```python
from build123d import *

# Parameters (mm, degrees)
SKETCH1_R           = 2.5
BOSS_EXTRUDE1_DEPTH = 8
CHAMFER1_SIZE       = 0.5
SKETCH2_R           = 1.5
CUT_EXTRUDE1_DEPTH  = 5


with BuildPart() as part:
    # Sketch1 → Boss-Extrude1 (new body)
    with BuildSketch(Plane.XY):
        with BuildLine():
            Line((-6, 15), (-6, 0))
            Line((-6, 0), (-25, 0))
            ThreePointArc((-25, 0), (0, -25), (25, 0))
            Line((25, 0), (6, 0))
            Line((6, 0), (6, 15))
            ThreePointArc((6, 15), (0, 21), (-6, 15))
        make_face()
        with Locations((0, 15)):
            Circle(SKETCH1_R, mode=Mode.SUBTRACT)
    extrude(amount=BOSS_EXTRUDE1_DEPTH)

    # Chamfer1
    chamfer1_edges = [part.edges().sort_by_distance(p)[0] for p in [
        (-2.5, 15, 8),
    ]]
    chamfer(chamfer1_edges, length=CHAMFER1_SIZE)

    # Sketch2 → Cut-Extrude1 (cut)
    with BuildSketch(Plane(origin=(0, 21, 0), x_dir=(1, 0, 0), z_dir=(0, 1, 0))):
        with Locations(Location((0, -4, 0), (0, 0, 270))):
            Circle(SKETCH2_R)
    extrude(amount=-CUT_EXTRUDE1_DEPTH, mode=Mode.SUBTRACT)


solid = part.part
```
For this review, take the finished solid that the model builds, in its own axes (mm). A direction names the side the tool comes from. Round coordinates to 2 decimals unless told otherwise and drop trailing zeros. Write each loop counter-clockwise with the first axis right and the second up, starting at its lowest first coordinate (ties: lowest second). Pieces come first, ordered by that corner, then holes. Notation, with made-up numbers: M 22.25,-14 L 60.25,-14 A21 cw 60.25,2 Z; hole C 4.5,-7 d10. An arc over 180 degrees is marked long. One line per item, written item: value. Start each with the question number.
(1) Insertion check: pin 1 (2 mm diameter, centred on x = 12.5, z = 5, fed in from +Y); pin 2 (4 mm diameter, centred on x = 0, z = 4, fed in from +Y); pin 3 (1.5 mm diameter, centred on y = 5.5, z = 5, fed in from +X); pin 4 (3 mm diameter, centred on y = -18.5, z = 1.5, fed in from -X). Each pin has a flat end and moves straight along its axis. Give the tip position at first contact, or say it passes through.
(2) The part is to be moulded in two halves that separate along Z. For faces 4 (the cylindrical face through (-0.575, 19.028, 5.386)), 5 (the flat face through (0, -7, 8)), 6 (the flat face through (-6, 8, 4)), 7 (the flat face through (0, -7, 0)), say which applies: released by +Z, released by -Z, zero draft, split by the parting line, or undercut.
(3) Machinability: for faces 1 (the flat face through (-15, 0, 4)), 2 (the cylindrical face through (-0.54, 12.56, 3.7)), 3 (the flat face through (16, 0, 4)), which of the approach directions +Z, -Z, +X, -X, +Y, -Y give a long, thin tool a straight path to every point of the face, cutting with its end or side? Answer none if there is none.
(4) We need section A-A (z = 4.5). Give the boundary of the cut face in (x, y).
(5) Wall thickness on line 1 (Y direction, x = 0, z = 6); line 2 (X direction, y = 13, z = 6.5); line 3 (Z direction, x = 0, y = 18.45): over which ranges is each line inside the solid? List them lowest first.
(6) We need section B-B (y = 6.5). Give the boundary of the cut face in (x, z), and give its area (3 significant figures).
(7) We need section C-C (x = 15). Give the boundary of the cut face in (y, z).
Result:
1. pin 1: y = 0
1. pin 2: y = 21
1. pin 3: x = 6
1. pin 4: x = -18.33
2. face 4: undercut
2. face 5: released by +Z
2. face 6: zero draft
2. face 7: released by -Z
3. face 1: +Z, -Z, -X, +Y
3. face 2: +Z, -Z
3. face 3: +Z, -Z, +X, +Y
4. outline: M -25,0 A25 ccw 25,0 L 6,0 L 6,15 A6 ccw 1.41,20.83 L 1.41,17.06 A2.5 cw long -1.41,17.06 L -1.41,20.83 A6 ccw -6,15 L -6,0 Z
5. line 1: -25 to 12.5, 17.5 to 21
5. line 2: -6 to -1.5, 1.5 to 6
5. line 3: 0 to 2.5, 5.5 to 8
6. outline: M -6,0 L 6,0 L 6,8 L -6,8 Z
6. area: 96.0 mm²
7. outline: M -20,0 L 0,0 L 0,8 L -20,8 Z
